Build history of the part. All positions in model axes, mm. A direction names the side the tool comes from. Coordinates: 2 decimals unless noted, no trailing zeros. Order: outer loops, then holes, each group sorted by start corner. A loop starts at its lowest first (then second) coordinate and runs counter-clockwise, first axis right, second up. Notation, with made-up numbers: (74.25, -15.5) - (90.25, -15.5) arc R18 cw to (90.25, 17.5) - close; hole circle Ø7 at (73, 53). An arc over 180 degrees is marked (long way). Write each question's results on one line, items separated by ' | '.
from build123d import *

# Parameters (mm, degrees)
F0_W     = 16
F0_H     = 16
F1_DEPTH = 10
F2_W     = 8
F2_H     = 10
F3_DEPTH = 10.001
F4_SIZE  = 1


with BuildPart() as f1:
    # F0 (on Front) → F1 (new body)
    with BuildSketch(Plane.XZ):
        with Locations((8, 8)):
            Rectangle(F0_W, F0_H)
    extrude(amount=F1_DEPTH)

    # F2 (on face) → F3 (cut, through all)
    with BuildSketch(Plane.XZ.offset(10)):
        with Locations((8, 5)):
            Rectangle(F2_W, F2_H)
    extrude(amount=-F3_DEPTH, mode=Mode.SUBTRACT)

    # F4
    f4_edges = [f1.edges().sort_by_distance(p)[0] for p in [
        (0, -5, 16),
        (16, -5, 16),
    ]]
    chamfer(f4_edges, length=F4_SIZE)


solid = f1.part
1. Tool access for faces 4 (the face through (12, -5, 5)), 5 (the face through (8, -10, 12)): list every direction of +Z, -Z, +X, -X, +Y, -Y with a clear straight run to the whole face (end or side of a thin tool).
Solved:
face 4: -Z, +Y, -Y | face 5: +Z, -Z, +X, -X, -Y
2. Band-saw the part on A-A on z = 1.75. Give the cut face in (x, y), then the cut area to 3 significant figures.
Solved:
outline: (0, -10) - (4, -10) - (4, 0) - (0, 0) - close; (12, -10) - (16, -10) - (16, 0) - (12, 0) - close | area: 80.0 mm2
3. Band-saw the part on B-B on y = -7. Give the cut face in (x, z).
Solved:
outline: (0, 0) - (4, 0) - (4, 10) - (12, 10) - (12, 0) - (16, 0) - (16, 15) - (15, 16) - (1, 16) - (0, 15) - close
4. Band-saw the part on D-D on x = 5. Give the cut face in (y, z), then the cut area to 3 significant figures.
Solved:
outline: (-10, 10) - (0, 10) - (0, 16) - (-10, 16) - close | area: 60.0 mm2
5. Probe line 1 (X direction, y = -5.25, z = 1.25); line 2 (Z direction, x = 11, y = -9). List the from-to ranges inside material, lowest first.
Solved:
line 1: x = 0 to 4, 12 to 16 | line 2: z = 10 to 16
6. Band-saw the part on C-C on z = 15.25. Give the cut face in (x, y).
Solved:
outline: (0.25, -10) - (15.75, -10) - (15.75, 0) - (0.25, 0) - close
7. Two-plate mould, pull along X, no slides. Class faces 1 (the face through (2, -5, 0)), 2 (the face through (8, -5, 10)), 3 (the face through (0, -5, 7)): +X half, -X half, draft (parallel to the pull), parting line (faces both ways), or undercut.
Solved:
face 1: draft | face 2: undercut | face 3: -X half
